```python
from build123d import *

# Parameters (mm, degrees)
SKETCH_1_W             = 40
SKETCH_1_H             = 30
EXTRUDE_1_DEPTH        = 4
SKETCH_3_W             = 40
SKETCH_3_H             = 4
EXTRUDE_2_DEPTH        = 65
FILLET_1_R             = 4
SKETCH_4_R             = 2.6
CUT_EXTRUDE_1_DEPTH    = 70.641941386
PATTERN_LINEAR_1_COUNT = 2
PATTERN_LINEAR_1_PITCH = 20
SKETCH_5_R             = 5
CUT_EXTRUDE_2_DEPTH    = 77.40026178
CHAMFER_1_SIZE         = 10
FILLET_2_R             = 5
FILLET_3_R             = 1


with BuildPart() as part:
    # 草圖1 → 填料-伸長1 (new body)
    with BuildSketch(Plane(origin=(0, 0, 0), x_dir=(1, 0, 0), z_dir=(0, 1, 0))):
        Rectangle(SKETCH_1_W, SKETCH_1_H)
    extrude(amount=EXTRUDE_1_DEPTH)

    # 草圖3 → 填料-伸長2 (add)
    with BuildSketch(Plane(origin=(0, 4, 0), x_dir=(1, 0, 0), z_dir=(0, 1, 0))):
        with Locations((0, 13)):
            Rectangle(SKETCH_3_W, SKETCH_3_H)
    extrude(amount=EXTRUDE_2_DEPTH)

    # 圓角1
    fillet_1_edges = [part.edges().sort_by_distance(p)[0] for p in [
        (0, 0, -15),
    ]]
    fillet(fillet_1_edges, radius=FILLET_1_R)

    # 草圖4 → 除料-伸長1 (cut, through all)
    with BuildSketch(Plane(origin=(0, 4, 0), x_dir=(1, 0, 0), z_dir=(0, 1, 0))):
        with Locations(Location((-10, 0, 0), (0, 0, 270))):
            Circle(SKETCH_4_R)
    cut_extrude_1 = extrude(amount=-CUT_EXTRUDE_1_DEPTH, mode=Mode.SUBTRACT)

    # 直線複製排列1: 除料-伸長1 ×2
    with Locations(*[(i * PATTERN_LINEAR_1_PITCH, 0, 0) for i in range(1, PATTERN_LINEAR_1_COUNT)]):
        add(cut_extrude_1, mode=Mode.SUBTRACT)

    # 草圖5 → 除料-伸長2 (cut, through all)
    with BuildSketch(Plane.XY.offset(-11)):
        with Locations((0, 49)):
            Circle(SKETCH_5_R)
    extrude(amount=-CUT_EXTRUDE_2_DEPTH, mode=Mode.SUBTRACT)

    # 導角1
    chamfer_1_edges = [part.edges().sort_by_distance(p)[0] for p in [
        (-20, 69, -13),
        (20, 69, -13),
        (20, 2, 15),
        (-20, 2, 15),
    ]]
    chamfer(chamfer_1_edges, length=CHAMFER_1_SIZE)

    # 圓角2
    fillet_2_edges = [part.edges().sort_by_distance(p)[0] for p in [
        (-10, 69, -13),
        (10, 69, -13),
        (20, 2, 5),
        (20, 59, -13),
        (-20, 2, 5),
        (-20, 59, -13),
        (10, 2, 15),
        (-10, 2, 15),
    ]]
    fillet(fillet_2_edges, radius=FILLET_2_R)

    # 圓角3
    fillet_3_edges = [part.edges().sort_by_distance(p)[0] for p in [
        (0, 4, -11),
    ]]
    fillet(fillet_3_edges, radius=FILLET_3_R)


solid = part.part
```
Can you work these out from the model? Positions are in its coordinate system, mm. Round coordinates to 2 decimals unless told otherwise and drop trailing zeros. Order: outer loops, then holes, each group sorted by start corner. A loop starts at its lowest first (then second) coordinate and runs counter-clockwise, first axis right, second up.
(1) We'd pull the mould along X, two halves only. Please class faces 1 (the face through (-12.54, 2.03, -0.56)), 2 (the face through (-19.63, 2.03, 4.82)), 3 (the face through (0, 69, -13)), 4 (the face through (9.82, 68.63, -13.03)): +X half, -X half, draft (parallel to the pull), parting line (faces both ways), or undercut.
Results are:
face 1: undercut
face 2: -X half
face 3: draft
face 4: +X half
(2) If we section it at A-A (z = 0): Please give me the cut outline in (x, y).
Results are:
outline: (-20, 0) - (-12.6, 0) - (-12.6, 4) - (-20, 4) - close; (-7.4, 0) - (7.4, 0) - (7.4, 4) - (-7.4, 4) - close; (12.6, 0) - (20, 0) - (20, 4) - (12.6, 4) - close
(3) I'm going to push flat-ended pins straight in: pin 1 (7.5 mm diameter, centred on x = -4, z = 8.5, fed in from +Y); pin 2 (8 mm diameter, centred on x = -6, y = 19, fed in from +Z). Where does each tip first touch, or does it pass through?
Results are:
pin 1: stops at y = 4
pin 2: stops at z = -11
(4) If we section it at D-D (x = 15.5): Please give me the cut outline in (y, z).
Results are:
outline: (0, -11) arc R4 ccw to (4, -15) - (63.5, -15) - (63.5, -11) - (5, -11) arc R1 cw to (4, -10) - (4, 9.5) - (0, 9.5) - close
(5) If I drill on L1, parallel to X at y = 3.15, z = 0; L2, parallel to Y at x = 3.5, z = 8.75; L3, parallel to Z at x = 13, y = 30, over which ranges is the centre line in solid material (lowest first)?
Results are:
L1: x = -20 to -12.6, -7.4 to 7.4, 12.6 to 20
L2: y = 0 to 4
L3: z = -15 to -11
(6) If we section it at C-C (y = 45): Please give me the cut outline in (x, z).
Results are:
outline: (-20, -15) - (-3, -15) - (-3, -11) - (-20, -11) - close; (3, -15) - (20, -15) - (20, -11) - (3, -11) - close
(7) If we section it at B-B (x = 0): Please give me the cut outline in (y, z).
Results are:
outline: (0, -11) arc R4 ccw to (4, -15) - (44, -15) - (44, -11) - (5, -11) arc R1 cw to (4, -10) - (4, 15) - (0, 15) - close; (54, -15) - (69, -15) - (69, -11) - (54, -11) - close
